Work out the finished part from the listing and answer in its coordinate system (mm). A direction names the side the tool comes from. Coordinates: 2 decimals unless noted, no trailing zeros. Order: outer loops, then holes, each group sorted by start corner. A loop starts at its lowest first (then second) coordinate and runs counter-clockwise, first axis right, second up. Notation, with made-up numbers: M 87,-16 L 146,-16 A11 cw 146,-10 Z; hole C 25,-31 d7. An arc over 180 degrees is marked long. Answer in a Markdown table with one row per item. Add a question column.
Item 1: The part is cut by section C-C (z = 0.75). State how many separate pieces and enclosed holes the cut face has, then the cut area to 3 significant figures.
Item 2: The mould has two halves that part along Y. Classify faces 4 (the face through (143.53, 50.91, 2.35)), 5 (the face through (144, 60, 2)), 6 (the face through (129, 40, 2)), 7 (the face through (141.86, 10.09, 2.35)): released by +Y, released by -Y, zero draft, split by the parting line, or undercut.
Item 3: Which of the six approach directions +Z, -Z, +X, -X, +Y, -Y give full straight-line access (tool end or side, diameter ignored) to faces 1 (the face through (10, 37, 3.3)), 2 (the face through (79, 20, 2)), 3 (the face through (13, 31, 2.3))?
Item 4: Flat-ended cylindrical pins translate along their axes: pin 1 Ø3 at (x, y) = (148, 44.5) entering from -Z; pin 2 Ø2.5 at (x, y) = (144, 38) entering from +Z. Find the tip coordinate at first contact, or state that the pin passes through.
Item 5: The part is cut by section B-B (y = 46). Write down the section's boundary in (x, z), then the cut area to 3 significant figures.
Item 6: The part is cut by section D-D (x = 15). Write down the section's boundary in (y, z), then the cut area to 3 significant figures.
Item 7: Consider line 1 (Y direction, x = 12.5, z = 1.8); line 2 (Y direction, x = 146.5, z = 1); line 3 (X direction, y = 45, z = 0.25). Determine where each line is inside the solid, lowest interval first. Write a range as from..to.
Item 8: The part is cut by section A-A (x = 79.5). Write down the section's boundary in (y, z), then the cut area to 3 significant figures.
from build123d import *

# Parameters (mm, degrees)
ESQUISSE1_W             = 159
ESQUISSE1_H             = 60
BOSS_EXTRU_1_DEPTH      = 4
ENL_V_START             = -4
ESQUISSE2_W             = 20.5
ESQUISSE2_H             = 4.8
ENL_V_MAT_EXTRU_1_DEPTH = 0.7
ESQUISSE3_R             = 5.25
ENL_V_MAT_EXTRU_2_DEPTH = 2.3
ESQUISSE4_W             = 99
ESQUISSE4_H             = 40
ENL_V_MAT_EXTRU_3_DEPTH = 4
ESQUISSE5_R             = 2
ENL_V_MAT_EXTRU_4_DEPTH = 4
CHANFREIN1_SIZE         = 3
CHANFREIN1_SIZE2        = 1.732050808


with BuildPart() as part:
    # Esquisse1 → Boss.-Extru.1 (new body)
    with BuildSketch(Plane.XY):
        with Locations((79.5, 30)):
            Rectangle(ESQUISSE1_W, ESQUISSE1_H)
    extrude(amount=BOSS_EXTRU_1_DEPTH)

    # Esquisse2 → Enlèv. mat.-Extru.1 (cut)
    with BuildSketch(Plane(origin=(0, 0, 0), x_dir=(-1, 0, 0), z_dir=(0, 0, -1)).offset(ENL_V_START)):
        with Locations((-10.25, 37.2)):
            Rectangle(ESQUISSE2_W, ESQUISSE2_H)
        with Locations((-148.75, 37.2)):
            Rectangle(ESQUISSE2_W, ESQUISSE2_H)
    extrude(amount=ENL_V_MAT_EXTRU_1_DEPTH, mode=Mode.SUBTRACT)

    # Esquisse3 → Enlèv. mat.-Extru.2 (cut)
    with BuildSketch(Plane(origin=(0, 0, 0), x_dir=(-1, 0, 0), z_dir=(0, 0, -1))):
        with Locations((-12.5, 31.187269084)):
            Circle(ESQUISSE3_R)
        with Locations((-12.5, 43.187269084)):
            Circle(ESQUISSE3_R)
        with Locations((-146.5, 31.204694992)):
            Circle(ESQUISSE3_R)
        with Locations((-146.5, 43.187269084)):
            Circle(ESQUISSE3_R)
    extrude(amount=-ENL_V_MAT_EXTRU_2_DEPTH, mode=Mode.SUBTRACT)

    # Esquisse4 → Enlèv. mat.-Extru.3 (cut)
    with BuildSketch(Plane.XY.offset(4)):
        with Locations((79.5, 40)):
            Rectangle(ESQUISSE4_W, ESQUISSE4_H)
    extrude(amount=-ENL_V_MAT_EXTRU_3_DEPTH, mode=Mode.SUBTRACT)

    # Esquisse5 → Enlèv. mat.-Extru.4 (cut)
    with BuildSketch(Plane.XY.offset(4)):
        with Locations((15, 10)):
            Circle(ESQUISSE5_R)
        with Locations((144, 10)):
            Circle(ESQUISSE5_R)
        with Locations((15, 53)):
            Circle(ESQUISSE5_R)
        with Locations((144, 53)):
            Circle(ESQUISSE5_R)
        with Locations((79.5, 10)):
            Circle(ESQUISSE5_R)
    extrude(amount=-ENL_V_MAT_EXTRU_4_DEPTH, mode=Mode.SUBTRACT)

    # Chanfrein1
    chanfrein1_edges = [part.edges().sort_by_distance(p)[0] for p in [
        (13, 10, 4),
        (142, 10, 4),
        (13, 53, 4),
        (142, 53, 4),
        (77.5, 10, 4),
    ]]
    chanfrein1_side = [part.faces().sort_by_distance(p)[0] for p in [
        (10.25, 33.100558915, 4),
    ]]
    chamfer(chanfrein1_edges, length=CHANFREIN1_SIZE, length2=CHANFREIN1_SIZE2, reference=chanfrein1_side[0])


solid = part.part
Reply:
| question | item | result |
|---|---|---|
| 1 | separate pieces | 1 |
| 1 | enclosed holes | 9 |
| 1 | area | 5,170 mm2 |
| 2 | face 4 | undercut |
| 2 | face 5 | released by +Y |
| 2 | face 6 | zero draft |
| 2 | face 7 | undercut |
| 3 | face 1 | +Z, -X |
| 3 | face 2 | +Z, -Z, +Y |
| 3 | face 3 | -Z |
| 4 | pin 1 | stops at z = 2.3 |
| 4 | pin 2 | stops at z = 3.3 |
| 5 | outline | M 0,0 L 8.07,0 L 8.07,2.3 L 16.93,2.3 L 16.93,0 L 30,0 L 30,4 L 0,4 Z; M 129,0 L 142.07,0 L 142.07,2.3 L 150.93,2.3 L 150.93,0 L 159,0 L 159,4 L 129,4 Z |
| 5 | area | 199 mm2 |
| 6 | outline | M 0,0 L 8,0 L 8,2.27 L 5,4 L 0,4 Z; M 12,0 L 26.57,0 L 26.57,2.3 L 35.8,2.3 L 35.8,0 L 38.57,0 L 38.57,2.3 L 47.8,2.3 L 47.8,0 L 51,0 L 51,2.27 L 48,4 L 39.6,4 L 39.6,3.3 L 34.8,3.3 L 34.8,4 L 15,4 L 12,2.27 Z; M 55,0 L 60,0 L 60,4 L 58,4 L 55,2.27 Z |
| 6 | area | 152 mm2 |
| 7 | line 1 | y = 0..25.94, 36.44..37.94, 48.44..60 |
| 7 | line 2 | y = 0..25.95, 36.45..37.94, 48.44..60 |
| 7 | line 3 | x = 0..7.57, 17.43..30, 129..141.57, 151.43..159 |
| 8 | outline | M 0,0 L 8,0 L 8,2.27 L 5,4 L 0,4 Z; M 12,0 L 20,0 L 20,4 L 15,4 L 12,2.27 Z |
| 8 | area | 58.8 mm2 |
